Answer from the drawing. Dimensions are ordinates in mm from the lowest x, y and z of the part. A direction names the side the tool comes from. Round coordinates to 2 decimals unless told otherwise and drop trailing zeros. Order: outer loops, then holes, each group sorted by start corner. A loop starts at its lowest first (then second) coordinate and runs counter-clockwise, first axis right, second up. Notation, with made-up numbers: (79.25, 6.25) - (83.25, 6.25) arc R26 cw to (83.25, 43.25) - close; hole circle Ø9 at (-23.75, 20.5). An arc over 180 degrees is marked (long way). One line per question, with ' | ' between items. Start each with the question number.
1) Straight lines are drawn through the part: line 1 (Y direction, x = 273, z = 64.5); line 2 (Z direction, x = 74.5, y = 72). For each, find the intervals that lie inside material, in ascending order. Write a range as from..to.
2) The mould has two halves that part along Y. Classify the marked faces 1, 2, 3 and 4: pulls with the +Y half, pulls with the -Y half, needs draft (parallel to the pull), parting line crosses it, or undercut.
3) The part is cut by section A-A, the plane z = 65. Give the vertices of the cut face in (x, y).
4) The part is cut by section C-C, the plane y = 268.5. Give the vertices of the cut face in (x, z).
5) The part is cut by section B-B, the plane x = 140. Give the vertices of the cut face in (y, z), plus the area to 3 significant figures.
6) For the marked faces 5 and 6, determine the directions among +Z, -Z, +X, -X, +Y, -Y from which every point of the face is accessible in a straight line to the end or side of a thin tool.
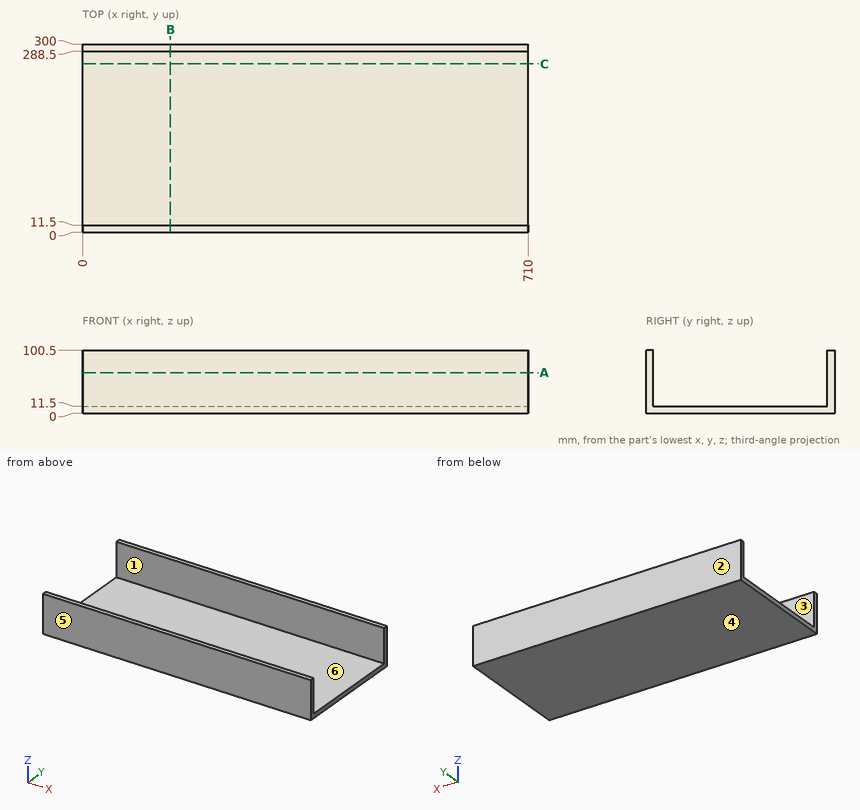
Values:
1) line 1: y = 0..11.5, 288.5..300 | line 2: z = 0..11.5
2) face 1: undercut | face 2: pulls with the +Y half | face 3: undercut | face 4: needs draft
3) outline: (0, 0) - (710, 0) - (710, 11.5) - (0, 11.5) - close; (0, 288.5) - (710, 288.5) - (710, 300) - (0, 300) - close
4) outline: (0, 0) - (710, 0) - (710, 11.5) - (0, 11.5) - close
5) outline: (0, 0) - (300, 0) - (300, 100.5) - (288.5, 100.5) - (288.5, 11.5) - (11.5, 11.5) - (11.5, 100.5) - (0, 100.5) - close | area: 5,500 mm^2
6) face 5: +Z, -Z, +X, -X, -Y | face 6: +Z, +X, -X
